from build123d import *

# Parameters (mm, degrees)
F0_W      = 35.56
F0_H      = 32.258
F1_DEPTH  = 12.7
F2_R      = 3.25
F3_DEPTH  = 32.259
F4_W      = 6.5
F4_H      = 6.5
F5_DEPTH  = 25.4
F6_W      = 42.65
F6_H      = 12.7
F7_DEPTH  = 19.05
F9_DEPTH  = 6.35
F10_W     = 14
F10_H     = 12.7
F11_DEPTH = 7.62
F12_R     = 5
F13_R     = 3.025
F14_DEPTH = 12.701
F15_R     = 3.025
F16_DEPTH = 4
F17_R     = 5
F19_DEPTH = 50.8
F20_W     = 15.96225
F20_H     = 9.625087
F21_DEPTH = 50.8


with BuildPart() as f1:
    # F0 (on Top) → F1 (new body, symmetric)
    with BuildSketch(Plane.XY):
        Rectangle(F0_W, F0_H)
        Polygon((11.43, 9.779), (11.43, -9.779), (-11.43, -9.779), (-11.43, 9.779), (-7.366, 9.779), (-7.366, 3.937), (4.826, 3.937), (4.826, 9.779), align=None, mode=Mode.SUBTRACT)
    extrude(amount=F1_DEPTH, both=True)

    # F2 (on face) → F3 (cut, through all)
    with BuildSketch(Plane.XZ.offset(16.129)):
        Circle(F2_R)
    extrude(amount=-F3_DEPTH, mode=Mode.SUBTRACT)

    # F4 (on face) → F5 (cut)
    with BuildSketch(Plane.XZ.offset(16.129)):
        Rectangle(F4_W, F4_H)
    extrude(amount=-F5_DEPTH, mode=Mode.SUBTRACT)

    # F6 (on face) → F7 (join)
    with BuildSketch(Plane(origin=(0, 0, -12.7), x_dir=(1, 0, 0), z_dir=(0, 0, -1))):
        with Locations((39.105, 9.779)):
            Rectangle(F6_W, F6_H)
    extrude(amount=-F7_DEPTH)

    # F8 (on face) → F9 (join)
    with BuildSketch(Plane.XZ.offset(16.129)):
        Polygon((17.78, 12.7), (17.78, 6.35), (43.18, 6.35), align=None)
    extrude(amount=-F9_DEPTH)

    # F10 (on face) → F11 (join)
    with BuildSketch(Plane(origin=(0, 0, -12.7), x_dir=(1, 0, 0), z_dir=(0, 0, -1))):
        with Locations((47.43, 9.779)):
            Rectangle(F10_W, F10_H)
    extrude(amount=F11_DEPTH)

    # F12
    f12_edges = [f1.edges().sort_by_distance(p)[0] for p in [
        (40.43, -9.779, -20.32),
        (54.43, -9.779, -20.32),
    ]]
    fillet(f12_edges, radius=F12_R)

    # F13 (on face) → F14 (cut, through all)
    with BuildSketch(Plane(origin=(0, -3.429, 0), x_dir=(-1, 0, 0), z_dir=(0, 1, 0))):
        with Locations((-47.43, -12.7)):
            Circle(F13_R)
    extrude(amount=-F14_DEPTH, mode=Mode.SUBTRACT)

    # F15 (on face) → F16 (cut)
    with BuildSketch(Plane(origin=(0, -3.429, 0), x_dir=(-1, 0, 0), z_dir=(0, 1, 0))):
        Polygon((-50.316751, -17.7), (-44.543249, -17.7), (-41.656497, -12.7), (-44.543249, -7.7), (-50.316751, -7.7), (-53.203503, -12.7), align=None)
        with Locations((-47.43, -12.7)):
            Circle(F15_R, mode=Mode.SUBTRACT)
    extrude(amount=-F16_DEPTH, mode=Mode.SUBTRACT)

    # F17
    f17_edges = [f1.edges().sort_by_distance(p)[0] for p in [
        (54.43, -9.779, -12.7),
        (40.43, -9.779, -12.7),
    ]]
    fillet(f17_edges, radius=F17_R)

    # F18 (on face) → F19 (cut)
    with BuildSketch(Plane.XY.offset(12.7)):
        Polygon((-17.78, 16.129), (-17.78, 8.001), (-11.43, 8.001), (-11.43, 9.779), (-7.366, 9.779), (-7.366, 8.001), (4.826, 8.001), (4.826, 9.779), (11.43, 9.779), (11.43, 8.001), (17.78, 8.001), (17.78, 16.129), align=None)
    extrude(amount=-F19_DEPTH, mode=Mode.SUBTRACT)

    # F20 (on face) → F21 (cut)
    with BuildSketch(Plane.XY.offset(12.7)):
        with Locations((0, 6.352621)):
            Rectangle(F20_W, F20_H)
    extrude(amount=-F21_DEPTH, mode=Mode.SUBTRACT)


solid = f1.part
Can you work these out from the model? Positions are in its coordinate system, mm. A direction names the side the tool comes from. Coordinates: 2 decimals unless noted, no trailing zeros. Write each loop counter-clockwise with the first axis right and the second up, starting at its lowest first coordinate (ties: lowest second). Pieces come first, ordered by that corner, then holes. Notation, with made-up numbers: (54.25, 0.5) -> (75.25, 0.5) arc R22 cw to (75.25, 32.5) -> close; hole circle Ø9 at (17.5, -27). An arc over 180 degrees is marked (long way). Write item = value, one per line.
(1) If I drill on probe 1 along X at (y, z) = (-4, -5.5); probe 2 along Z at (x, y) = (47.43, -13.5) (3 decimals); probe 3 along Z at (x, y) = (45.5, -6), over which ranges is the centre line in solid material (lowest first)?
Verdict:
probe_1 = -17.78 to -11.43, 11.43 to 60.43
probe_2 = -20.32 to -15.725, -9.675 to 6.35
probe_3 = -20.32 to -17.7, -7.7 to 6.35
(2) On a 3-axis mill with a long thin cutter (end or side, diameter ignored), from which of +Z, -Z, +X, -X, +Y, -Y can I reach the whole of each face in a straight line? I mean faces 4 (the face through (51.78, -5.401, -15.165)), 5 (the face through (9, -12, -12.7)), 6 (the face through (11.43, -1, 0)). Say none if no direction works.
Verdict:
face_4 = +Y
face_5 = -Z, -X, +Y, -Y
face_6 = +Z, -Z, +Y
(3) For pin 1 (1.5 mm diameter, centred on x = -2, z = 5.5, fed in from +Y); pin 2 (4.5 mm diameter, centred on x = 46.5, y = -5.5, fed in from +Z); pin 3 (6 mm diameter, centred on x = 16.5, y = 5.5, fed in from -Z), each with a flat end and sliding along its axis, tell me the tip position at first contact or that it passes through.
Verdict:
pin_1 = -9.78
pin_2 = 6.35
pin_3 = -12.7
(4) Imagine slicing it at A-A (y = 3). Please give me the cut outline in (x, z), and give its area (3 significant figures).
Verdict:
outline = (-17.78, -12.7) -> (-11.43, -12.7) -> (-11.43, 12.7) -> (-17.78, 12.7) -> close; (11.43, -12.7) -> (17.78, -12.7) -> (17.78, 12.7) -> (11.43, 12.7) -> close
area = 323 mm^2
(5) Imagine slicing it at C-C (z = -11.5). Please give me the cut outline in (x, y), and give its area (3 significant figures).
Verdict:
outline = (-17.78, -16.13) -> (44.65, -16.13) -> (44.65, -7.43) -> (42.35, -7.43) -> (42.35, -3.43) -> (17.78, -3.43) -> (17.78, 8) -> (11.43, 8) -> (11.43, -9.78) -> (-11.43, -9.78) -> (-11.43, 8) -> (-17.78, 8) -> close; (50.21, -16.13) -> (60.43, -16.13) -> (60.43, -3.43) -> (52.51, -3.43) -> (52.51, -7.43) -> (50.21, -7.43) -> close
area = 904 mm^2
(6) Imagine slicing it at B-B (x = 47.43). Please give me the cut outline in (y, z) (3 decimals), and give its area (3 significant figures).
Verdict:
outline = (-16.129, -20.32) -> (-3.429, -20.32) -> (-3.429, -17.7) -> (-7.429, -17.7) -> (-7.429, -15.725) -> (-16.129, -15.725) -> close; (-16.129, -9.675) -> (-7.429, -9.675) -> (-7.429, -7.7) -> (-3.429, -7.7) -> (-3.429, 6.35) -> (-16.129, 6.35) -> close
area = 246 mm^2
(7) Thinking about a two-plate mould opening in Z: for faces 1 (the face through (42.307, -9.868, -19.225)), 2 (the face through (17.78, 1, 0)), 3 (the face through (51.74, -5.401, -10.165)), which applies, +Z half, -Z half, draft (parallel to the pull), parting line (faces both ways), or undercut?
Verdict:
face_1 = -Z half
face_2 = draft
face_3 = undercut
(8) Imagine slicing it at D-D (y = -6). State how many separate pieces and enclosed holes the cut face has, and give its area (3 significant figures).
Verdict:
separate_pieces = 2
enclosed_holes = 1
area = 1,150 mm^2
